```python
from build123d import *

# Parameters (mm, degrees)
SKETCH3_W                = 91
SKETCH3_H                = 87.244293111
BOSS_EXTRUDE1_DEPTH      = 35
BOSS_EXTRUDE1_DEPTH_BACK = 5
SKETCH2_W                = 85
SKETCH2_H                = 81.244293111
CUT_EXTRUDE1_DEPTH       = 41
CUT_EXTRUDE2_REACH       = 89.244
SKETCH5_R                = 7
SKETCH5_W                = 18
SKETCH5_H                = 14.87


with BuildPart() as part:
    # Sketch3 → Boss-Extrude1 (new body, two sides)
    with BuildSketch(Plane.XY) as boss_extrude1_sk:
        with Locations((40.316463084, 38.577850393)):
            Rectangle(SKETCH3_W, SKETCH3_H)
    extrude(amount=BOSS_EXTRUDE1_DEPTH)
    extrude(boss_extrude1_sk.sketch, amount=-BOSS_EXTRUDE1_DEPTH_BACK)

    # Sketch2 → Cut-Extrude1 (cut)
    with BuildSketch(Plane.XY):
        with Locations((40.316463084, 38.577850393)):
            Rectangle(SKETCH2_W, SKETCH2_H)
    extrude(amount=CUT_EXTRUDE1_DEPTH, mode=Mode.SUBTRACT)

    # Sketch5 → Cut-Extrude2 (cut, up to next)
    with BuildSketch(Plane.XZ.offset(5.044296163), mode=Mode.PRIVATE) as cut_extrude2_sk1:
        with Locations((72.107645341, 23.62352)):
            Circle(SKETCH5_R)
    cut_extrude2_tool1 = extrude(cut_extrude2_sk1.sketch, amount=-CUT_EXTRUDE2_REACH, mode=Mode.PRIVATE) & part.part
    add(cut_extrude2_tool1.solids().sort_by_distance((72.107645, -5.044296, 23.62352))[0], mode=Mode.SUBTRACT)
    # Sketch5 → Cut-Extrude2 (cut, up to next)
    with BuildSketch(Plane.XZ.offset(5.044296163), mode=Mode.PRIVATE) as cut_extrude2_sk2:
        with Locations((33.464005425, 23.62352)):
            Rectangle(SKETCH5_W, SKETCH5_H)
    cut_extrude2_tool2 = extrude(cut_extrude2_sk2.sketch, amount=-CUT_EXTRUDE2_REACH, mode=Mode.PRIVATE) & part.part
    add(cut_extrude2_tool2.solids().sort_by_distance((33.464005, -5.044296, 23.62352))[0], mode=Mode.SUBTRACT)


solid = part.part
```
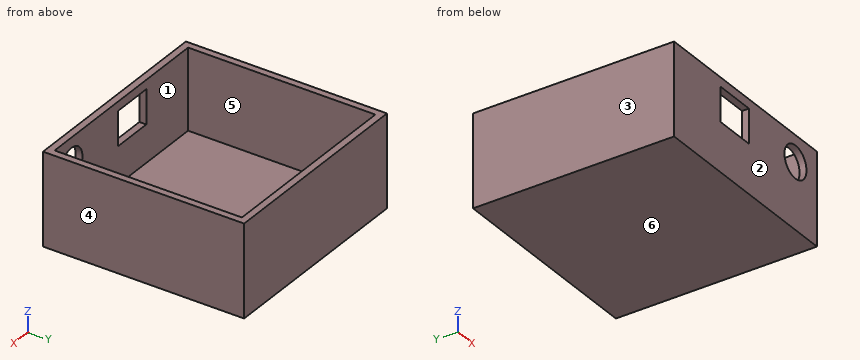
Geometry check sheet. Reference: the model listing, model coordinates, mm. Face numbers are marked on the shaded views. A direction names the side the tool comes from. Give positions to 0.01 mm unless a question says otherwise; leave off trailing zeros. Order: outer loops, then holes, each group sorted by start corner. A loop starts at its lowest first (then second) coordinate and runs counter-clockwise, first axis right, second up. Notation, with made-up numbers: (76, 77.25) - (120, 77.25) arc R19 cw to (120, 101.25) - close; hole circle Ø3 at (56, 35). An arc over 180 degrees is marked (long way). Write item = value, one per line. Start each with the question number.
1) Access from +Z, -Z, +X, -X, +Y, -Y to the whole of each face (thin tool, end or side, straight path). Record for the marked faces 1 and 2.
2) Draft check along X on the marked faces 3, 4, 5 and 6. Enter one of: released by +X, released by -X, zero draft, split by the parting line, or undercut.
3) Gauge pin test, flat end, axial feed: pin 1 Ø1 at (x, y) = (19.5, 6) entering from +Z. Record the tip position at first contact, or that the pin passes through.
4) Section check B-B (z = 15). Enter the section's corners in (x, y).
5) Scan lines: L1, parallel to Y at x = 59, z = 27; L2, parallel to X at y = 0.5, z = 17; L3, parallel to Z at x = 23, y = 21. Record each from-to range of solid material in increasing order.
6) Section check D-D (z = 29.5). Enter the section's corners in (x, y).
7) Section check A-A (x = 33). Enter the section's corners in (y, z), then the cut area to 3 significant figures.
8) Section check C-C (y = 51.5). Enter the section's corners in (x, z), then the cut area to 3 significant figures.
Geometry check:
q1.face_1 = +Z
q1.face_2 = +Z, -Z, +X, -X, -Y
q2.face_3 = released by -X
q2.face_4 = released by +X
q2.face_5 = undercut
q2.face_6 = zero draft
q3.pin_1 = 0
q4.outline = (-5.18, -5.04) - (85.82, -5.04) - (85.82, 82.2) - (-5.18, 82.2) - close; hole (-2.18, -2.04) - (82.82, -2.04) - (82.82, 79.2) - (-2.18, 79.2) - close
q5.L1 = -5.04 to -2.04, 79.2 to 82.2
q5.L2 = -5.18 to -2.18, 82.82 to 85.82
q5.L3 = -5 to 0
q6.outline = (-5.18, -5.04) - (24.46, -5.04) - (24.46, -2.04) - (-2.18, -2.04) - (-2.18, 79.2) - (82.82, 79.2) - (82.82, -2.04) - (75.91, -2.04) - (75.91, -5.04) - (85.82, -5.04) - (85.82, 82.2) - (-5.18, 82.2) - close; (42.46, -5.04) - (68.3, -5.04) - (68.3, -2.04) - (42.46, -2.04) - close
q7.outline = (-5.04, -5) - (82.2, -5) - (82.2, 35) - (79.2, 35) - (79.2, 0) - (-2.04, 0) - (-2.04, 16.19) - (-5.04, 16.19) - close; (-5.04, 31.06) - (-2.04, 31.06) - (-2.04, 35) - (-5.04, 35) - close
q7.area = 602 mm2
q8.outline = (-5.18, -5) - (85.82, -5) - (85.82, 35) - (82.82, 35) - (82.82, 0) - (-2.18, 0) - (-2.18, 35) - (-5.18, 35) - close
q8.area = 665 mm2
